Geometry check sheet. Reference: the model listing, model coordinates, mm. Face numbers are marked on the shaded views. Round coordinates to 2 decimals unless told otherwise and drop trailing zeros. Write each loop counter-clockwise with the first axis right and the second up, starting at its lowest first coordinate (ties: lowest second). Pieces come first, ordered by that corner, then holes.
Item 1: Draft check along X on the marked faces 1, 2 and 3. Enter one of: pulls with the +X half, pulls with the -X half, needs draft (parallel to the pull), parting line crosses it, or undercut.
Item 2: Cross-section at D-D (x = -5.5). Enter the section's corners in (y, z), then the cut area to 3 significant figures.
Item 3: Cross-section at B-B (x = 0). Enter the section's corners in (y, z), then the cut area to 3 significant figures.
Item 4: Cross-section at C-C (y = 4.5). Enter the section's corners in (x, z), then the cut area to 3 significant figures.
Item 5: Scan lines: probe 1 along X at (y, z) = (0.95, 0); probe 2 along Y at (x, z) = (-13.5, -15.5); probe 3 along X at (y, z) = (5, 10). Record each from-to range of solid material in increasing order.
Item 6: Cross-section at A-A (z = 0). Enter the section's corners in (x, y), then the cut area to 3 significant figures.
Item 7: Depth check by flat-ended pin: P1, Ø6, axis at x = -15.5, z = -3.5, coming from the +Y side. Enter the tip coordinate at first touch or a pass-through.
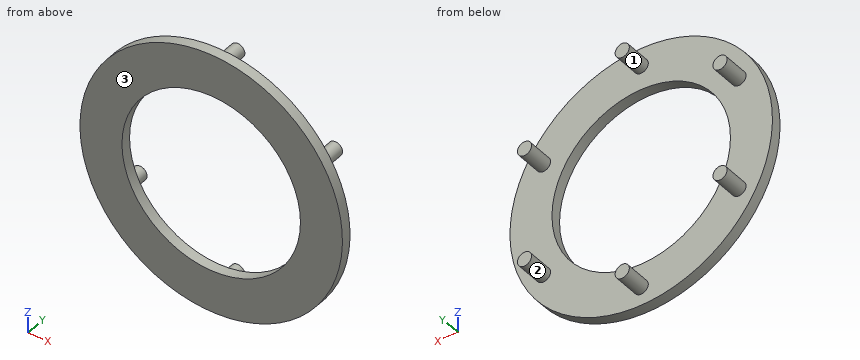
from build123d import *

# Parameters (mm, degrees)
SKETCH1_R           = 25
SKETCH1_R_2         = 1.35
SKETCH1_R_3         = 17
BOSS_EXTRUDE1_DEPTH = 2
SKETCH1_3_R         = 1.35
BOSS_EXTRUDE2_DEPTH = 7


with BuildPart() as part:
    # Sketch1 → Boss-Extrude1 (new body)
    with BuildSketch(Plane(origin=(0, 0, 0), x_dir=(1, 0, 0), z_dir=(0, 1, 0))):
        with Locations(Location((0, 0, 0), (0, 0, 270))):
            Circle(SKETCH1_R)
        with Locations(Location((0, 21.5, 0), (0, 0, 270))):
            Circle(SKETCH1_R_2, mode=Mode.SUBTRACT)
        with Locations(Location((18.619546181, 10.75, 0), (0, 0, 270))):
            Circle(SKETCH1_R_2, mode=Mode.SUBTRACT)
        with Locations(Location((18.619546181, -10.75, 0), (0, 0, 270))):
            Circle(SKETCH1_R_2, mode=Mode.SUBTRACT)
        with Locations(Location((0, -21.5, 0), (0, 0, 270))):
            Circle(SKETCH1_R_2, mode=Mode.SUBTRACT)
        with Locations(Location((-18.619546181, -10.75, 0), (0, 0, 270))):
            Circle(SKETCH1_R_2, mode=Mode.SUBTRACT)
        with Locations(Location((-18.619546181, 10.75, 0), (0, 0, 270))):
            Circle(SKETCH1_R_2, mode=Mode.SUBTRACT)
        with Locations(Location((0, 0, 0), (0, 0, 270))):
            Circle(SKETCH1_R_3, mode=Mode.SUBTRACT)
    extrude(amount=BOSS_EXTRUDE1_DEPTH)

    # Sketch1_3 → Boss-Extrude2 (add)
    with BuildSketch(Plane(origin=(0, 0, 0), x_dir=(1, 0, 0), z_dir=(0, 1, 0))):
        with Locations(Location((-18.619546181, -10.75, 0), (0, 0, 270))):
            Circle(SKETCH1_3_R)
        with Locations(Location((-18.619546181, 10.75, 0), (0, 0, 270))):
            Circle(SKETCH1_3_R)
        with Locations(Location((0, 21.5, 0), (0, 0, 270))):
            Circle(SKETCH1_3_R)
        with Locations(Location((18.619546181, 10.75, 0), (0, 0, 270))):
            Circle(SKETCH1_3_R)
        with Locations(Location((18.619546181, -10.75, 0), (0, 0, 270))):
            Circle(SKETCH1_3_R)
        with Locations(Location((0, -21.5, 0), (0, 0, 270))):
            Circle(SKETCH1_3_R)
    extrude(amount=BOSS_EXTRUDE2_DEPTH)


solid = part.part
Resolved:
1. face 1: parting line crosses it
1. face 2: undercut
1. face 3: needs draft
2. outline: (0, -24.39) - (2, -24.39) - (2, -16.09) - (0, -16.09) - close; (0, 16.09) - (2, 16.09) - (2, 24.39) - (0, 24.39) - close
2. area: 33.2 mm2
3. outline: (0, -25) - (2, -25) - (2, -22.85) - (7, -22.85) - (7, -20.15) - (2, -20.15) - (2, -17) - (0, -17) - close; (0, 17) - (2, 17) - (2, 20.15) - (7, 20.15) - (7, 22.85) - (2, 22.85) - (2, 25) - (0, 25) - close
3. area: 59.0 mm2
4. outline: circle Ø2.7 at (-18.62, -10.75); circle Ø2.7 at (-18.62, 10.75); circle Ø2.7 at (0, -21.5); circle Ø2.7 at (0, 21.5); circle Ø2.7 at (18.62, -10.75); circle Ø2.7 at (18.62, 10.75)
4. area: 34.4 mm2
5. probe 1: x = -25 to -17, 17 to 25
5. probe 2: y = 0 to 2
5. probe 3: x = -19.74 to -17.5, 17.5 to 19.74
6. outline: (-25, 0) - (-17, 0) - (-17, 2) - (-25, 2) - close; (17, 0) - (25, 0) - (25, 2) - (17, 2) - close
6. area: 32.0 mm2
7. P1: stops at y = 2
